Could you check a few things on this model? Use its own coordinates, in mm. Face numbers are marked on the shaded views. Round coordinates to 2 decimals unless told otherwise and drop trailing zeros. Loops run counter-clockwise (first coordinate to the right, second up) from the corner with the lowest first, then second, coordinate; pieces in that order, holes last. Notation, with made-up numbers: M 65,11.25 L 103,11.25 A35 cw 103,50.25 Z; hole C -6,-25 d10. An arc over 180 degrees is marked long. Return JSON: item names as keys, results as strings. Group by question number.
```python
from build123d import *

# Parameters (mm, degrees)
BASPROSKE_W        = 5
BASPROSKE_H        = 6
TOOTHCUT_DEPTH     = 10.848857802
TEETHCUTS_COUNT    = 10
TEETHCUTS_ANGLE    = 324
BORSKE_R           = 1.5
BORE_DEPTH         = 50.0000508
SKETCH1_R          = 3
CUT_EXTRUDE1_DEPTH = 3
SCALE1_SCALE       = 0.95
SKETCH2_R          = 1.75
CUT_EXTRUDE2_DEPTH = 9.38856389


with BuildPart() as part:
    # BasProSke → Base-Revolve (revolve)
    with BuildSketch(Plane(origin=(0, 0, 0), x_dir=(1, 0, 0), z_dir=(0, 1, 0)), mode=Mode.PRIVATE) as base_revolve_sk:
        with Locations((2.5, 3)):
            Rectangle(BASPROSKE_W, BASPROSKE_H)
    revolve(base_revolve_sk.sketch.rotate(Axis((-10, 0, 0), (1, 0, 0)), 180), axis=Axis((-10, 0, 0), (1, 0, 0)))

    # TooCutSke → ToothCut (cut, through all)
    with BuildSketch(Plane(origin=(0, 0, 0), x_dir=(0, 0, -1), z_dir=(1, 0, 0))):
        with BuildLine():
            ThreePointArc((0.59278292, 3.701838653), (0, 3.749), (-0.59278292, 3.701838653))
            ThreePointArc((-0.59278292, 3.701838653), (-0.846593509, 4.924114224), (-1.775771316, 5.757784417))
            ThreePointArc((-1.775771316, 5.757784417), (0, 6.0254), (1.775771316, 5.757784417))
            ThreePointArc((1.775771316, 5.757784417), (0.846593509, 4.924114224), (0.59278292, 3.701838653))
        make_face()
    toothcut = extrude(amount=TOOTHCUT_DEPTH, mode=Mode.SUBTRACT)

    # TeethCuts: ToothCut ×10 about axis
    teethcuts_axis = Axis((-10, 0, 0), (1, 0, 0))
    for i in range(1, TEETHCUTS_COUNT):
        add(toothcut.rotate(teethcuts_axis, i * TEETHCUTS_ANGLE / (TEETHCUTS_COUNT - 1)), mode=Mode.SUBTRACT)

    # BorSke → Bore (cut, symmetric)
    with BuildSketch(Plane(origin=(0, 0, 0), x_dir=(0, 0, -1), z_dir=(1, 0, 0))):
        with Locations(Location((0, 0, 0), (0, 0, 180))):
            Circle(BORSKE_R)
    extrude(amount=BORE_DEPTH, both=True, mode=Mode.SUBTRACT)

    # Sketch1 → Cut-Extrude1 (cut)
    with BuildSketch(Plane(origin=(5, 0, 0), x_dir=(0, 0, -1), z_dir=(1, 0, 0))):
        Circle(SKETCH1_R)
    extrude(amount=-CUT_EXTRUDE1_DEPTH, mode=Mode.SUBTRACT)


with BuildPart() as part_1:
    # Scale1: scaled about (2.255821785, 0, 0)
    add(part.part.scale(SCALE1_SCALE).moved(Location((0.112791089, 0, 0))))

    # Sketch2 → Cut-Extrude2 (cut, through all)
    with BuildSketch(Plane(origin=(2.012791089, 0, 0), x_dir=(0, 0, -1), z_dir=(1, 0, 0))):
        Circle(SKETCH2_R)
    extrude(amount=-CUT_EXTRUDE2_DEPTH, mode=Mode.SUBTRACT)


solid = part_1.part
```
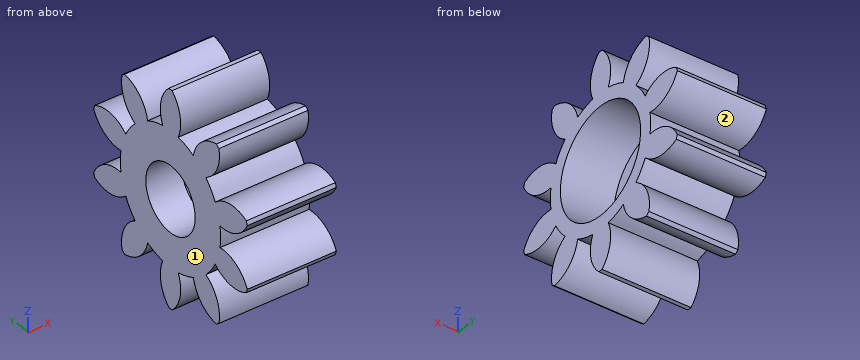
1. If we section it at B-B, the plane y = -3: Please give me the cut outline in (x, z), then the cut area to 3 significant figures.
2. I'm going to push flat-ended pins straight in: pin 1 Ø5.5 at (y, z) = (0, 0) entering from +X; pin 2 Ø2 at (x, y) = (3, -3) entering from -Z; pin 3 Ø2 at (x, z) = (4.5, -3.5) entering from +Y. Where does each tip first touch, or does it pass through?
3. I need wall thicknesses on probe 1 along Y at (x, z) = (3.85, 0); probe 2 along Y at (x, z) = (0.85, 0); probe 3 along Z at (x, y) = (3.3, 3.25). Which ranges of each line are inside material? Lowest first, please.
4. If we section it at C-C, the plane y = 4.75: Please give me the cut outline in (x, z).
5. If we section it at A-A, the plane z = 0: Please give me the cut outline in (x, y).
6. We'd pull the mould along Z, two halves only. Please class the marked faces 1 and 2: +Z half, -Z half, draft (parallel to the pull), parting line (faces both ways), or undercut.
Geometry results:
{
 "1": {"outline": "M 0.11,-4.63 L 4.86,-4.63 L 4.86,-2.92 L 0.11,-2.92 Z; M 0.11,-1.92 L 4.86,-1.92 L 4.86,1.92 L 0.11,1.92 Z; M 0.11,2.92 L 4.86,2.92 L 4.86,4.63 L 0.11,4.63 Z", "area": "34.5 mm^2"},
 "2": {"pin 1": "x = 2.01", "pin 2": "z = -4.68", "pin 3": "y = 3.48"},
 "3": {"probe 1": "-3.56 to -2.85, 2.85 to 3.56", "probe 2": "-3.56 to -1.75, 1.75 to 3.56", "probe 3": "-4.68 to -3.27, -1.68 to 1.68, 3.27 to 4.68"},
 "4": {"outline": "M 0.11,-2.09 L 4.86,-2.09 L 4.86,-0.85 L 0.11,-0.85 Z; M 0.11,0.85 L 4.86,0.85 L 4.86,2.09 L 0.11,2.09 Z"},
 "5": {"outline": "M 0.11,-3.56 L 4.86,-3.56 L 4.86,-2.85 L 2.01,-2.85 L 2.01,-1.75 L 0.11,-1.75 Z; M 0.11,1.75 L 2.01,1.75 L 2.01,2.85 L 4.86,2.85 L 4.86,3.56 L 0.11,3.56 Z"},
 "6": {"face 1": "draft", "face 2": "undercut"}
}
